from build123d import *

# Parameters (mm, degrees)
BOSS_EXTRU_3_DEPTH       = 88
ESQUISSE4_W              = 68
ESQUISSE4_H              = 76.5
ENL_V_MAT_EXTRU_1_DEPTH  = 236.459258684
ENL_V_MAT_EXTRU_2_DEPTH  = 68
ENL_V_MAT_EXTRU_5_REACH  = 245.615
ESQUISSE6_W              = 150.690647389
ESQUISSE6_H              = 20
BOSS_EXTRU_5_DEPTH       = 20
ESQUISSE14_W             = 40
ESQUISSE14_H             = 40
ENL_V_MAT_EXTRU_6_DEPTH  = 236.459258684
BOSS_EXTRU_8_DEPTH       = 40
ENL_V_MAT_EXTRU_7_DEPTH  = 236.984242059
ESQUISSE27_W             = 169
ESQUISSE27_H             = 5
BOSS_EXTRU_9_DEPTH       = 45.5
BOSS_EXTRU_10_REACH      = 258.45
ESQUISSE28_R             = 5
ENL_V_MAT_EXTRU_9_DEPTH  = 45.5
BOSS_EXTRU_12_DEPTH      = 17.5
ENL_V_MAT_EXTRU_10_REACH = 248.129
BOSS_EXTRU_13_REACH      = 258.45
ESQUISSE34_R             = 5
BOSS_EXTRU_14_DEPTH      = 17.5
ESQUISSE36_W             = 20
ESQUISSE36_H             = 20
ENL_V_MAT_EXTRU_11_DEPTH = 256.967405152
ESQUISSE42_R             = 5
ENL_V_MAT_EXTRU_16_DEPTH = 10
ESQUISSE43_R             = 5
ENL_V_MAT_EXTRU_17_DEPTH = 10


with BuildPart() as part:
    # Esquisse1 → Boss.-Extru.3 (new body)
    with BuildSketch(Plane(origin=(0, 0, 0), x_dir=(1, 0, 0), z_dir=(0, 1, 0))):
        Polygon((193, 20), (6, 48.25), (-44, 48.25), (-44, -48.25), (6, -48.25), (193, -20), (213, -20), (213, 20), align=None)
    extrude(amount=BOSS_EXTRU_3_DEPTH)

    # Esquisse4 → Enlèv. mat.-Extru.1 (cut, through all)
    with BuildSketch(Plane(origin=(0, 88, 0), x_dir=(1, 0, 0), z_dir=(0, 1, 0))):
        Rectangle(ESQUISSE4_W, ESQUISSE4_H)
    extrude(amount=-ENL_V_MAT_EXTRU_1_DEPTH, mode=Mode.SUBTRACT)

    # Esquisse5 → Enlèv. mat.-Extru.2 (cut)
    with BuildSketch(Plane(origin=(0, 88, 0), x_dir=(1, 0, 0), z_dir=(0, 1, 0))):
        Polygon((193, 20), (173, 20), (173, 2.5), (44, 2.5), (44, 42.509358289), align=None)
        Polygon((173, -20), (193, -20), (44, -42.509358289), (44, -2.5), (173, -2.5), align=None)
    extrude(amount=-ENL_V_MAT_EXTRU_2_DEPTH, mode=Mode.SUBTRACT)

    # Enlèv. mat.-Extru.5: up to this plane
    enl_v_mat_extru_5_end = Plane(origin=(173, 20, 2.5), z_dir=(0, 0, -1))
    # Esquisse6 → Enlèv. mat.-Extru.5 (cut, up to the surface)
    with BuildSketch(Plane(origin=(7.260340781, 0, 48.059600925), x_dir=(0.9887806747234926, 0, -0.14937462064673088), z_dir=(0.14937462064673088, 0, 0.9887806747234927)), mode=Mode.PRIVATE) as enl_v_mat_extru_5_sk1:
        with Locations((112.501854115, 10)):
            Rectangle(ESQUISSE6_W, ESQUISSE6_H)
    enl_v_mat_extru_5_tool1 = split(extrude(enl_v_mat_extru_5_sk1.sketch, amount=-ENL_V_MAT_EXTRU_5_REACH, mode=Mode.PRIVATE), bisect_by=enl_v_mat_extru_5_end, keep=Keep.BOTH, mode=Mode.PRIVATE)
    add(enl_v_mat_extru_5_tool1.solids().sort_by_distance((118.5, 10, 31.254679))[0], mode=Mode.SUBTRACT)

    # Esquisse11 → Boss.-Extru.5 (add)
    with BuildSketch(Plane.XZ.offset(-20)):
        Polygon((37.955805499, 2.5), (44, 2.5), (44, 42.509358289), align=None)
    extrude(amount=BOSS_EXTRU_5_DEPTH)

    # Esquisse14 → Enlèv. mat.-Extru.6 (cut, through all)
    with BuildSketch(Plane(origin=(0, 88, 0), x_dir=(1, 0, 0), z_dir=(0, 1, 0))):
        with Locations((193, 0)):
            Rectangle(ESQUISSE14_W, ESQUISSE14_H)
    extrude(amount=-ENL_V_MAT_EXTRU_6_DEPTH, mode=Mode.SUBTRACT)

    # Esquisse22 → Boss.-Extru.8 (add)
    with BuildSketch(Plane(origin=(173, 0, 0), x_dir=(0, 0, -1), z_dir=(1, 0, 0))):
        Polygon((-2.5, 0), (20, 0), (20, 20), (2.5, 20), (2.5, 88), (-2.5, 88), align=None)
    extrude(amount=BOSS_EXTRU_8_DEPTH)

    # Esquisse23 → Enlèv. mat.-Extru.7 (cut, through all)
    with BuildSketch(Plane.XY.offset(2.5)):
        with BuildLine():
            Line((213, 0), (213, 40))
            Line((213, 40), (193, 40))
            Line((193, 40), (159, 40))
            Line((159, 40), (134.047464579, 40))
            ThreePointArc((134.047464579, 40), (133, 39.767782693), (132.14881397, 39.114644681))
            Line((132.14881397, 39.114644681), (103.122598553, 4.522548178))
            ThreePointArc((103.122598553, 4.522548178), (98.774593016, 1.186206186), (93.423962687, 0))
            Line((93.423962687, 0), (213, 0))
        make_face()
    extrude(amount=-ENL_V_MAT_EXTRU_7_DEPTH, mode=Mode.SUBTRACT)

    # Esquisse27 → Boss.-Extru.9 (add)
    with BuildSketch(Plane(origin=(0, 88, 0), x_dir=(1, 0, 0), z_dir=(0, 1, 0))):
        with Locations((128.5, 0)):
            Rectangle(ESQUISSE27_W, ESQUISSE27_H)
    extrude(amount=BOSS_EXTRU_9_DEPTH)

    # Boss.-Extru.10: up to this plane
    boss_extru_10_end = Plane(origin=(7.260340781, 88, 48.059600925), z_dir=(-0.14937462064673085, 0, -0.9887806747234926))
    # Esquisse28 → Boss.-Extru.10 (add, up to the surface)
    with BuildSketch(Plane.XY.offset(2.5), mode=Mode.PRIVATE) as boss_extru_10_sk1:
        with BuildLine():
            Line((103.122598553, 4.522548178), (132.14881397, 39.114644681))
            ThreePointArc((132.14881397, 39.114644681), (133, 39.767782693), (134.047464579, 40))
            Line((134.047464579, 40), (159, 40))
            Line((159, 40), (193, 40))
            Line((193, 40), (193, 60))
            Line((193, 60), (173, 60))
            Line((173, 60), (163, 60))
            ThreePointArc((163, 60), (155.928932188, 57.071067812), (153, 50))
            Line((153, 50), (153, 46))
            Line((153, 46), (134.047464579, 46))
            ThreePointArc((134.047464579, 46), (130.46429043, 45.205629416), (127.552547311, 42.971370339))
            Line((127.552547311, 42.971370339), (98.526331894, 8.379273836))
            ThreePointArc((98.526331894, 8.379273836), (96.238883445, 6.624052908), (93.423962687, 6))
            Line((93.423962687, 6), (69, 6))
            Line((69, 6), (69, 10))
            ThreePointArc((69, 10), (66.071067812, 17.071067812), (59, 20))
            Line((59, 20), (44, 20))
            Line((44, 20), (44, 0))
            Line((44, 0), (63, 0))
            Line((63, 0), (93.423962687, 0))
            ThreePointArc((93.423962687, 0), (98.774593016, 1.186206186), (103.122598553, 4.522548178))
        make_face()
        with Locations((59, 10)):
            Circle(ESQUISSE28_R, mode=Mode.SUBTRACT)
        with Locations((163, 50)):
            Circle(ESQUISSE28_R, mode=Mode.SUBTRACT)
    boss_extru_10_tool1 = split(extrude(boss_extru_10_sk1.sketch, amount=BOSS_EXTRU_10_REACH, mode=Mode.PRIVATE), bisect_by=boss_extru_10_end, keep=Keep.BOTH, mode=Mode.PRIVATE)
    add(boss_extru_10_tool1.solids().sort_by_distance((124.30992, 30.316725, 2.5))[0])

    # Esquisse29 → Enlèv. mat.-Extru.9 (cut)
    with BuildSketch(Plane.XY.offset(2.5)):
        with BuildLine():
            ThreePointArc((145.939599002, 130.613536933), (147.768845256, 132.309522469), (149.96093833, 133.5))
            Line((149.96093833, 133.5), (44, 133.5))
            Line((44, 133.5), (44, 88))
            Line((44, 88), (105.519519296, 88))
            ThreePointArc((105.519519296, 88), (109.745701914, 88.93692213), (113.179963727, 91.572123903))
            Line((113.179963727, 91.572123903), (145.939599002, 130.613536933))
        make_face()
    extrude(amount=-ENL_V_MAT_EXTRU_9_DEPTH, mode=Mode.SUBTRACT)

    # Esquisse31 → Boss.-Extru.12 (add)
    with BuildSketch(Plane.XY.offset(2.5)):
        Polygon((213, 133.5), (173, 133.5), (173, 60), (193, 60), (193, 40), (213, 40), align=None)
    extrude(amount=BOSS_EXTRU_12_DEPTH)

    # Esquisse33 → Enlèv. mat.-Extru.10 (cut, up to next)
    with BuildSketch(Plane(origin=(0, 20, 0), x_dir=(1, 0, 0), z_dir=(0, 1, 0)), mode=Mode.PRIVATE) as enl_v_mat_extru_10_sk1:
        Polygon((44, 42.509358289), (44, 2.5), (116.109722668, 2.5), (116.109722668, 31.615777191), align=None)
    enl_v_mat_extru_10_tool1 = extrude(enl_v_mat_extru_10_sk1.sketch, amount=-ENL_V_MAT_EXTRU_10_REACH, mode=Mode.PRIVATE) & part.part
    add(enl_v_mat_extru_10_tool1.solids().sort_by_distance((78.160873, 20, -19.924346))[0], mode=Mode.SUBTRACT)

    # Boss.-Extru.13: up to this plane
    boss_extru_13_end = Plane(origin=(7.260340781, 88, -48.059600925), z_dir=(0.14937462064673085, 0, -0.9887806747234926))
    # Esquisse34 → Boss.-Extru.13 (add, up to the surface)
    with BuildSketch(Plane(origin=(0, 0, -2.5), x_dir=(-1, 0, 0), z_dir=(0, 0, -1)), mode=Mode.PRIVATE) as boss_extru_13_sk1:
        with BuildLine():
            Line((-44, 0), (-44, 20))
            Line((-44, 20), (-59, 20))
            ThreePointArc((-59, 20), (-66.071067812, 17.071067812), (-69, 10))
            Line((-69, 10), (-69, 6))
            Line((-69, 6), (-93.423962687, 6))
            ThreePointArc((-93.423962687, 6), (-96.238883445, 6.624052908), (-98.526331894, 8.379273836))
            Line((-98.526331894, 8.379273836), (-127.552547311, 42.971370339))
            ThreePointArc((-127.552547311, 42.971370339), (-130.46429043, 45.205629416), (-134.047464579, 46))
            Line((-134.047464579, 46), (-153, 46))
            Line((-153, 46), (-153, 50))
            ThreePointArc((-153, 50), (-155.928932188, 57.071067812), (-163, 60))
            Line((-163, 60), (-173, 60))
            Line((-173, 60), (-193, 60))
            Line((-193, 60), (-193, 40))
            Line((-193, 40), (-159, 40))
            Line((-159, 40), (-134.047464579, 40))
            ThreePointArc((-134.047464579, 40), (-133, 39.767782693), (-132.14881397, 39.114644681))
            Line((-132.14881397, 39.114644681), (-103.122598553, 4.522548178))
            ThreePointArc((-103.122598553, 4.522548178), (-98.774593016, 1.186206186), (-93.423962687, 0))
            Line((-93.423962687, 0), (-63, 0))
            Line((-63, 0), (-44, 0))
        make_face()
        with Locations(Location((-163, 50, 0), (0, 0, 180))):
            Circle(ESQUISSE34_R, mode=Mode.SUBTRACT)
        with Locations(Location((-59, 10, 0), (0, 0, 180))):
            Circle(ESQUISSE34_R, mode=Mode.SUBTRACT)
    boss_extru_13_tool1 = split(extrude(boss_extru_13_sk1.sketch, amount=BOSS_EXTRU_13_REACH, mode=Mode.PRIVATE), bisect_by=boss_extru_13_end, keep=Keep.BOTH, mode=Mode.PRIVATE)
    add(boss_extru_13_tool1.solids().sort_by_distance((124.30992, 30.316725, -2.5))[0])

    # Esquisse35 → Boss.-Extru.14 (add)
    with BuildSketch(Plane(origin=(0, 0, -2.5), x_dir=(-1, 0, 0), z_dir=(0, 0, -1))):
        Polygon((-173, 60), (-173, 133.5), (-213, 133.5), (-213, 40), (-193, 40), (-193, 60), align=None)
    extrude(amount=BOSS_EXTRU_14_DEPTH)

    # Esquisse36 → Enlèv. mat.-Extru.11 (cut, through all)
    with BuildSketch(Plane(origin=(0, 133.5, 0), x_dir=(1, 0, 0), z_dir=(0, 1, 0))):
        with Locations((193, 0)):
            Rectangle(ESQUISSE36_W, ESQUISSE36_H)
    extrude(amount=-ENL_V_MAT_EXTRU_11_DEPTH, mode=Mode.SUBTRACT)

    # Esquisse42 → Enlèv. mat.-Extru.16 (cut)
    with BuildSketch(Plane(origin=(0, 0, -2.5), x_dir=(-1, 0, 0), z_dir=(0, 0, -1))):
        with Locations(Location((-59, 10, 0), (0, 0, 180))):
            Circle(ESQUISSE42_R)
    extrude(amount=-ENL_V_MAT_EXTRU_16_DEPTH, mode=Mode.SUBTRACT)

    # Esquisse43 → Enlèv. mat.-Extru.17 (cut)
    with BuildSketch(Plane(origin=(0, 0, -2.5), x_dir=(-1, 0, 0), z_dir=(0, 0, -1))):
        with Locations(Location((-163, 50, 0), (0, 0, 180))):
            Circle(ESQUISSE43_R)
    extrude(amount=-ENL_V_MAT_EXTRU_17_DEPTH, mode=Mode.SUBTRACT)


solid = part.part
Build history of the part. All positions in model axes, mm. A direction names the side the tool comes from. Round coordinates to 2 decimals unless told otherwise and drop trailing zeros. Write each loop counter-clockwise with the first axis right and the second up, starting at its lowest first coordinate (ties: lowest second). Pieces come first, ordered by that corner, then holes. Notation, with made-up numbers: M -39.75,22.5 L -26.75,22.5 A34 cw -26.75,52.5 Z; hole C 31.5,74 d1. An arc over 180 degrees is marked long. Answer in a Markdown table with one row per item.
1. Saw through at D-D (y = 23.5). List the corners of the cut face in (x, z), and give its area (3 significant figures).
Geometry check:
| item | result |
|---|---|
| outline | M -44,-48.25 L 6,-48.25 L 44,-42.51 L 44,-2.5 L 111.21,-2.5 L 111.21,-32.36 L 119.05,-31.17 L 119.05,31.17 L 111.21,32.36 L 111.21,2.5 L 44,2.5 L 44,42.51 L 6,48.25 L -44,48.25 Z; hole M -34,-38.25 L 34,-38.25 L 34,38.25 L -34,38.25 Z |
| area | 3,910 mm2 |
2. Flat gauge pins, fed straight in: P1, Ø5, axis at x = 71, y = 58.5, coming from the +Z side; P2, Ø5.5, axis at x = 147, z = -14, coming from the +Y side; P3, Ø8, axis at x = 59, y = 10, coming from the +Z side; P4, Ø5, axis at x = 126.5, z = 2, coming from the -Y side. Where does each tip first touch, or does it go through?
Geometry check:
| item | result |
|---|---|
| P1 | z = 2.5 |
| P2 | y = 46 |
| P3 | through |
| P4 | y = 29.4 |
3. Which spindle directions (+Z, -Z, +X, -X, +Y, -Y) get a long thin tool onto all of the face, cutting with end or side? Do faces 1 (the face through (0, 45, -38.25)), 2 (the face through (113.243, 25.917, 18.164)), 3 (the face through (96.202, 6.607, -18.544)). Say none if no direction does.
Geometry check:
| item | result |
|---|---|
| face 1 | +Y, -Y |
| face 2 | +Z, +Y |
| face 3 | -Z, +Y |
4. Mould opens along X. For faces 4 (the face through (112.836, 25.433, -18.164)), 5 (the face through (193, 87, 20)), 6 (the face through (-44, 43, -1)) say: +X half, -X half, draft (parallel to the pull), parting line (faces both ways), or undercut.
Geometry check:
| item | result |
|---|---|
| face 4 | undercut |
| face 5 | draft |
| face 6 | -X half |
5. Probe L1, parallel to X at y = 50, z = 0; L2, parallel to Y at x = 59, z = -21.5; L3, parallel to Y at x = 59, z = 1.4. List the from-to ranges inside material, lowest first. Write a range as [from, to].
Geometry check:
| item | result |
|---|---|
| L1 | [-44, -34], [34, 158], [168, 183], [203, 213] |
| L2 | [0, 5], [15, 20] |
| L3 | [0, 5], [15, 88] |
6. Saw through at A-A (x = 196.5). List the corners of the cut face in (y, z), and give its area (3 significant figures).
Geometry check:
| item | result |
|---|---|
| outline | M 40,-20 L 133.5,-20 L 133.5,-10 L 40,-10 Z; M 40,10 L 133.5,10 L 133.5,20 L 40,20 Z |
| area | 1,870 mm2 |
7. Saw through at C-C (y = 95). List the corners of the cut face in (x, z).
Geometry check:
| item | result |
|---|---|
| outline | M 116.06,-2.5 L 173,-2.5 L 173,-20 L 213,-20 L 213,20 L 173,20 L 173,2.5 L 116.06,2.5 Z; hole M 183,-10 L 203,-10 L 203,10 L 183,10 Z |
8. Saw through at B-B (y = 70). List the corners of the cut face in (x, z), and give its area (3 significant figures).
Geometry check:
| item | result |
|---|---|
| outline | M -44,-48.25 L 6,-48.25 L 44,-42.51 L 44,-2.5 L 173,-2.5 L 173,-20 L 213,-20 L 213,20 L 173,20 L 173,2.5 L 44,2.5 L 44,42.51 L 6,48.25 L -44,48.25 Z; hole M -34,-38.25 L 34,-38.25 L 34,38.25 L -34,38.25 Z; hole M 183,-10 L 203,-10 L 203,10 L 183,10 Z |
| area | 4,920 mm2 |
